Could you check a few things on this model? Use its own coordinates, in mm. Face numbers are marked on the shaded views. A direction names the side the tool comes from. Give positions to 0.01 mm unless a question says otherwise; leave off trailing zeros. Order: outer loops, then holes, each group sorted by start corner. A loop starts at its lowest first (then second) coordinate and runs counter-clockwise, first axis right, second up. Notation, with made-up numbers: M 68,9.25 L 87,9.25 A9 cw 87,15.25 Z; hole C 63,33 d7. An arc over 180 degrees is marked long. Use a Markdown table: item, result. Add a question column.
Item 1: For the marked faces 1, 2, 3 and 4, which set-ups out of +Z, -Z, +X, -X, +Y, -Y let a thin tool reach every point of the face, with its end or its side?
Item 2: I'm going to push flat-ended pins straight in: pin 1 Ø4.5 at (y, z) = (-15.5, 15.5) entering from +X; pin 2 Ø3 at (y, z) = (5.5, 27) entering from +X; pin 3 Ø7.5 at (x, z) = (25, 23.5) entering from -Y. Where does each tip first touch, or does it pass through?
Item 3: Suppose I cut it at C-C on z = 8. Write out the boundary of the cut face in (x, y), plus the area to 3 significant figures.
Item 4: Suppose I cut it at A-A on z = 29.5. Write out the boundary of the cut face in (x, y).
Item 5: Suppose I cut it at B-B on y = 15. Write out the boundary of the cut face in (x, z) (3 decimals).
Item 6: If I drill on L1, parallel to Z at x = 0, y = -12.5; L2, parallel to Y at x = 0, z = 15.75; L3, parallel to Z at x = 0, y = 21, over which ranges is the centre line in solid material (lowest first)? Write a range as from..to.
Item 7: Suppose I cut it at D-D on x = -4. Write out the boundary of the cut face in (y, z), plus the area to 3 significant figures.
Item 8: If we mould it in two halves opening along X, with no side actions, what happens to the marked faces 5, 6, 7 and 8? For each: released by +X, released by -X, zero draft, split by the parting line, or undercut.
Autodesk Inventor part; units mm, degrees
ref_plane "YZ Plane" through (0, 0, 0) normal (1, 0, 0) x (0, 1, 0)
ref_plane "XZ Plane" through (0, 0, 0) normal (0, 1, 0) x (-1, 0, 0)
ref_plane "XY Plane" through (0, 0, 0) normal (0, 0, 1) x (1, 0, 0)
sketch "Sketch1" plane through (0, 0, 0) normal (0, 0, 1) x (1, 0, 0)
  line L0 (-32, 23) -> (32, 23)
  line L1 (32, 23) -> (32, -13)
  line L2 (7.75, -23) -> (-7.75, -23)
  line L3 (-32, -13) -> (-32, 23)
  line L4 (7.75, -13) -> (32, -13)
  line L5 (7.75, -23) -> (7.75, -13)
  line L6 (-32, -13) -> (-7.75, -13)
  line L7 (-7.75, -13) -> (-7.75, -23)
  point P0 (0, 0)
  dimension "d2" = 32
  dimension "d3" = 23
extrude "Extrusion1" add sketch "Sketch1" along normal blind 10
sketch "Sketch2" plane through (0, 0, 10) normal (0, 0, 1) x (1, 0, 0)
  line L0 (-32, -13) -> (-7.75, -13)
  line L1 (-32, -13) -> (-32, -5)
  line L2 (-32, 23) -> (-32, -13)
  line L3 (-32, -5) -> (-29, -5)
  line L4 (32, -13) -> (32, 23)
  line L5 (32, -9) -> (32, -5)
  line L6 (32, -5) -> (29, -5)
  line L7 (-7.75, -13) -> (-7.75, -23)
  line L8 (7.75, -13) -> (32, -13)
  arc A0 (12.8, 16.6) -> (-12.8, 16.6) centre (0, 7) ccw
  line L9 (-29, -5) -> (-12.8, 16.6)
  line L10 (29, -5) -> (12.8, 16.6)
  line L11 (-32, -13) -> (-7.75, -13)
  line L12 (-7.75, -23) -> (7.75, -23)
  line L13 (-7.75, -23) -> (7.75, -23)
  line L14 (7.75, -23) -> (7.75, -13)
  line L15 (7.75, -23) -> (7.75, -13)
  line L16 (7.75, -13) -> (32, -13)
  line L17 (32, -5) -> (32, -13)
  point P0 (0, 0)
  dimension "d15" = 32
extrude "Extrusion2" add sketch "Sketch2" along normal blind 22
sketch "Sketch3" plane through (0, 0, 32) normal (0, 0, 1) x (1, 0, 0)
  line L0 (-32, -5) -> (-32, -13)
  circle A0 centre (0, 7) radius 6
  point P0 (0, 0)
extrude "Extrusion3" cut sketch "Sketch3" against normal up to surface (22 mm away)
sketch "Sketch5" plane through (-32, 23, 0) normal (0, 1, 0) x (1, 0, 0)
  line L0 (32, 0) -> (32, -20)
  circle A0 centre (32, -20) radius 5
  circle A1 centre (32, -20) radius 2.875
  dimension "d22" = 20
  dimension "d23" = 10
  dimension "d36" = 5.75
extrude "Extrusion4" cut sketch "Sketch5" against normal blind 12 contours A1
extrude "Extrusion5" cut sketch "Sketch5" against normal blind 4 contours A1 | A0
sketch "Sketch6" plane through (-7.75, -23, 0) normal (0, -1, 0) x (1, 0, 0)
  point P0 (7.75, 0)
sketch "Sketch7" plane through (-7.75, -23, 0) normal (0, -1, 0) x (1, 0, 0)
  line L0 (0, 32) -> (15.5, 32)
  circle A0 centre (7.75, 24) radius 3
  circle A1 centre (7.75, 8) radius 3
  point P0 (7.75, 0)
  dimension "d31" = 6
  dimension "d32" = 6
extrude "Extrusion6" cut sketch "Sketch7" against normal blind 18
fillet "Fillet1" radius 3 2 edges at (29, -5, 21) (-29, -5, 21)
sketch "Sketch8" plane through (0, 0, 32) normal (0, 0, 1) x (1, 0, 0)
  line L0 (-7.75, -22) -> (7.75, -22)
  line L1 (7.75, -22) -> (7.75, -23)
  line L2 (7.75, -23) -> (-7.75, -23)
  line L3 (-7.75, -23) -> (-7.75, -22)
  line L4 (-7.75, -23) -> (7.75, -23)
  line L5 (-7.75, -13) -> (-7.75, -23)
  line L6 (7.75, -23) -> (7.75, -13)
  point P0 (0, 0)
  dimension "d37" = 1
extrude "Extrusion7" cut sketch "Sketch8" against normal through all
properties part number "Pieza4_corredera_LAASR" material "Steel, Carbon"
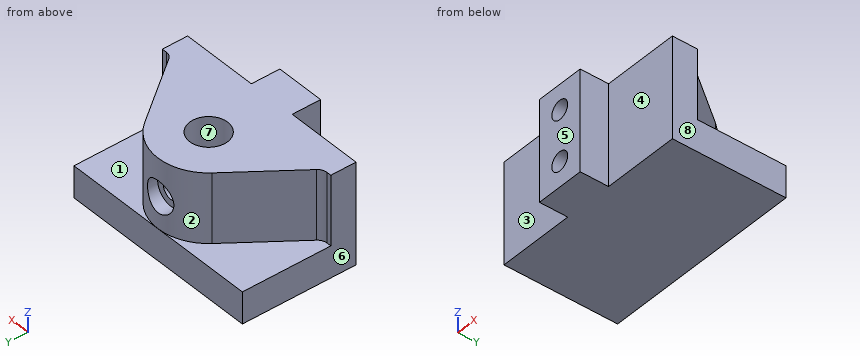
Findings below:
| question | item | result |
|---|---|---|
| 1 | face 1 | +Z, +X, +Y |
| 1 | face 2 | +Z, +Y |
| 1 | face 3 | +Z, -Z, -X, -Y |
| 1 | face 4 | +Z, -Z, +X, -Y |
| 2 | pin 1 | stops at x = 7.75 |
| 2 | pin 2 | stops at x = 22.25 |
| 2 | pin 3 | stops at y = -13 |
| 3 | outline | M -32,-13 L -7.75,-13 L -7.75,-22 L -3,-22 L -3,-5 L 3,-5 L 3,-22 L 7.75,-22 L 7.75,-13 L 32,-13 L 32,23 L -32,23 Z |
| 3 | area | 2,340 mm^2 |
| 4 | outline | M -32,-13 L -7.75,-13 L -7.75,-22 L 7.75,-22 L 7.75,-13 L 32,-13 L 32,-5 L 30.5,-5 A3 cw 28.1,-3.8 L 12.8,16.6 A16 ccw -12.8,16.6 L -28.1,-3.8 A3 cw -30.5,-5 L -32,-5 Z; hole C 0,7 d12 |
| 5 | outline | M -32,0 L 32,0 L 32,10 L 14,10 L 14,32 L -14,32 L -14,10 L -32,10 Z; hole C 0,20 d5.75 |
| 6 | L1 | z = 0..5, 11..21, 27..32 |
| 6 | L2 | y = -22..1, 13..19 |
| 6 | L3 | z = 0..15, 25..32 |
| 7 | outline | M -22,0 L 23,0 L 23,10 L 22.49,10 L 22.49,17 L 19,17 L 19,23 L 22.49,23 L 22.49,32 L 11.47,32 L 11.47,10 L 2.53,10 L 2.53,32 L -22,32 Z |
| 7 | area | 1,210 mm^2 |
| 8 | face 5 | zero draft |
| 8 | face 6 | released by -X |
| 8 | face 7 | undercut |
| 8 | face 8 | released by +X |
